Here's how the part is built. I have some questions about the finished solid (model axes, mm). Face numbers are marked on the shaded views. A direction names the side the tool comes from. Give positions to 0.01 mm unless a question says otherwise; leave off trailing zeros. Loops run counter-clockwise (first coordinate to the right, second up) from the corner with the lowest first, then second, coordinate; pieces in that order, holes last.
Q1. If we section it at A-A (z = -87.5): Please give me the cut outline in (x, y) (1 decimal).
Q2. For the marked faces 1 and 2, which set-ups out of +Z, -Z, +X, -X, +Y, -Y let a thin tool reach every point of the face, with its end or its side?
Q3. If we section it at C-C (z = -125.5): Please give me the cut outline in (x, y), plus the area to 3 significant figures.
Q4. Will this pin go through, and if not, where does the flat tip stop? P1, Ø1.5, axis at x = 190, y = 42, coming from the -Z side.
Q5. If we section it at D-D (x = 54): Please give me the cut outline in (y, z).
Q6. If we section it at B-B (y = 70): Please give me the cut outline in (x, z) (1 decimal).
Q7. I need wall thicknesses on line 1 (X direction, y = 116.5, z = -38.5); line 2 (Y direction, x = 44.5, z = -109); line 3 (Y direction, x = 7, z = -87.5). Which ranges of each line are inside material? Lowest first, please.
Q8. We'd pull the mould along X, two halves only. Please class the marked faces 3, 4, 5 and 6: +X half, -X half, draft (parallel to the pull), parting line (faces both ways), or undercut.
from build123d import *

# Parameters (mm, degrees)
SKETCH1_W           = 262
SKETCH1_H           = 150
BOSS_EXTRUDE1_DEPTH = 20
BOSS_EXTRUDE2_DEPTH = 100
SKETCH3_R           = 14.2875
CUT_EXTRUDE1_DEPTH  = 11
SKETCH4_R           = 15.875
CUT_EXTRUDE2_DEPTH  = 11
SKETCH5_W           = 262
SKETCH5_H           = 150
BOSS_EXTRUDE4_DEPTH = 10


with BuildPart() as part:
    # Sketch1 → Boss-Extrude1 (new body)
    with BuildSketch(Plane(origin=(0, 0, 0), x_dir=(1, 0, 0), z_dir=(0, 1, 0))):
        with Locations((131, 75)):
            Rectangle(SKETCH1_W, SKETCH1_H)
    extrude(amount=BOSS_EXTRUDE1_DEPTH)

    # Sketch2 → Boss-Extrude2 (add)
    with BuildSketch(Plane(origin=(0, 20, 0), x_dir=(1, 0, 0), z_dir=(0, 1, 0))):
        Polygon((0, 0), (262, 0), (262, 150), (252, 150), (252, 10), (10, 10), (10, 150), (0, 150), align=None)
    extrude(amount=BOSS_EXTRUDE2_DEPTH)

    # Sketch3 → Cut-Extrude1 (cut, through all)
    with BuildSketch(Plane(origin=(10, 0, 0), x_dir=(0, 0, -1), z_dir=(1, 0, 0))):
        with Locations((87.5, 70)):
            Circle(SKETCH3_R)
    extrude(amount=-CUT_EXTRUDE1_DEPTH, mode=Mode.SUBTRACT)

    # Sketch4 → Cut-Extrude2 (cut, through all)
    with BuildSketch(Plane(origin=(252, 0, 0), x_dir=(0, 0, -1), z_dir=(1, 0, 0))):
        with Locations((87.5, 70)):
            Circle(SKETCH4_R)
    extrude(amount=CUT_EXTRUDE2_DEPTH, mode=Mode.SUBTRACT)

    # Sketch5 → Boss-Extrude4 (add)
    with BuildSketch(Plane(origin=(0, 120, 0), x_dir=(1, 0, 0), z_dir=(0, 1, 0))):
        with Locations((131, 75)):
            Rectangle(SKETCH5_W, SKETCH5_H)
    extrude(amount=BOSS_EXTRUDE4_DEPTH)


solid = part.part
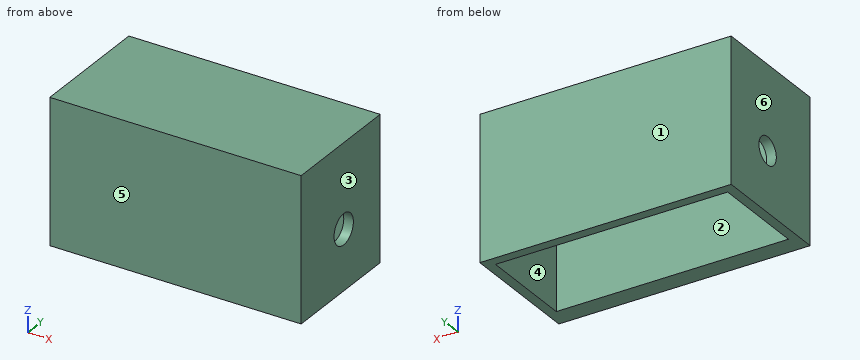
Check sheet entries:
1. outline: (0, 0) - (262, 0) - (262, 54.1) - (252, 54.1) - (252, 20) - (10, 20) - (10, 55.7) - (0, 55.7) - close; (0, 84.3) - (10, 84.3) - (10, 120) - (252, 120) - (252, 85.9) - (262, 85.9) - (262, 130) - (0, 130) - close
2. face 1: +Z, -Z, +X, -X, +Y
2. face 2: -Z
3. outline: (0, 0) - (262, 0) - (262, 130) - (0, 130) - close; hole (10, 20) - (252, 20) - (252, 120) - (10, 120) - close
3. area: 9,860 mm2
4. P1: stops at z = -10
5. outline: (0, -150) - (20, -150) - (20, -10) - (120, -10) - (120, -150) - (130, -150) - (130, 0) - (0, 0) - close
6. outline: (0, -150) - (10, -150) - (10, -101.8) - (0, -101.8) - close; (0, -73.2) - (10, -73.2) - (10, -10) - (252, -10) - (252, -71.6) - (262, -71.6) - (262, 0) - (0, 0) - close; (252, -150) - (262, -150) - (262, -103.4) - (252, -103.4) - close
7. line 1: x = 0 to 10, 252 to 262
7. line 2: y = 0 to 20, 120 to 130
7. line 3: y = 0 to 55.71, 84.29 to 130
8. face 3: +X half
8. face 4: undercut
8. face 5: draft
8. face 6: -X half
